The listing builds one solid part. Answer for the finished solid, in the listing's coordinates (mm). A direction names the side the tool comes from. Round coordinates to 2 decimals unless told otherwise and drop trailing zeros. Order: outer loops, then holes, each group sorted by start corner. A loop starts at its lowest first (then second) coordinate and runs counter-clockwise, first axis right, second up. Notation, with made-up numbers: (9, 18.25) - (16, 18.25) arc R8 cw to (16, 27.25) - close; hole circle Ø5 at (24, 80.25). An arc over 180 degrees is marked (long way). One line per item, written item: value. Start each with the question number.
1. A tool of negligible diameter and unlimited length cuts with its end or side. For faces 1 (the cylindrical face through (3.75, 66.42, 4.53)), 2 (the flat face through (30, 70, 2)), 3 (the flat face through (11, 72, 3)), from which of +Z, -Z, +X, -X, +Y, -Y can it reach the whole face along a straight path? Write none if from no direction.
2. Section C-C, the plane x = 10 is taken. Give the vertices of the cut face in (y, z).
3. Section B-B, the plane x = 23.5 is taken. Give the vertices of the cut face in (y, z), then the cut area to 3 significant figures.
4. Section A-A, the plane y = 60 is taken. Give the vertices of the cut face in (x, z).
5. For a pull along Y with two mould halves and no side action, classify faces 4 (the flat face through (1, 66, 2)), 5 (the flat face through (22, 24, 5)), 6 (the flat face through (22, 131, 3)) as released by +Y, released by -Y, zero draft, split by the parting line, or undercut.
6. Straight lines are drawn through the part: line 1 (X direction, y = 39, z = 0.75); line 2 (Y direction, x = 32, z = 3.25); line 3 (Y direction, x = 24, z = 3.75). For each, find the intervals that lie inside material, in ascending order.
7. Flat-ended cylindrical pins translate along their axes: P1, Ø0.6, axis at y = 118, z = 4.5, coming from the -X side; P2, Ø12, axis at x = 32, y = 62, coming from the +Z side; P3, Ø5, axis at x = 27, y = 85, coming from the +Z side; P4, Ø1.6, axis at y = 24.5, z = 4, coming from the -X side. Find the tip coordinate at first contact, or state that the pin passes through.
from build123d import *

# Parameters (mm, degrees)
F0_W      = 45
F0_H      = 131
F1_DEPTH  = 2
F2_W      = 40.5
F2_H      = 131
F3_DEPTH  = 5
F5_W      = 35
F5_H      = 100
F6_DEPTH  = 4
F7_W      = 5
F7_H      = 100
F8_DEPTH  = 2
F4_W      = 15
F4_H      = 90
F9_DEPTH  = 7.001
F10_R     = 1.5
F11_DEPTH = 131.001


with BuildPart() as f1:
    # F0 (on Top) → F1 (new body)
    with BuildSketch(Plane.XY):
        with Locations((22.5, 65.5)):
            Rectangle(F0_W, F0_H)
    extrude(amount=F1_DEPTH)

    # F2 (on face) → F3 (join)
    with BuildSketch(Plane.XY.offset(2)):
        with Locations((22.5, 65.5)):
            Rectangle(F2_W, F2_H)
    extrude(amount=F3_DEPTH)

    # F5 (on face) → F6 (cut)
    with BuildSketch(Plane.XY.offset(7)):
        with Locations((22.5, 71)):
            Rectangle(F5_W, F5_H)
    extrude(amount=-F6_DEPTH, mode=Mode.SUBTRACT)

    # F7 (on face) → F8 (join)
    with BuildSketch(Plane.XY.offset(3)):
        with Locations((22.5, 71)):
            Rectangle(F7_W, F7_H)
    extrude(amount=F8_DEPTH)

    # F4 (on face) → F9 (cut, through all)
    with BuildSketch(Plane.XY.offset(7)):
        with Locations((22.5, 71)):
            Rectangle(F4_W, F4_H)
    extrude(amount=-F9_DEPTH, mode=Mode.SUBTRACT)

    # F10 (on face) → F11 (cut, through all)
    with BuildSketch(Plane(origin=(0, 131, 0), x_dir=(-1, 0, 0), z_dir=(0, 1, 0))):
        with Locations((-42.75, 4.5)):
            Circle(F10_R)
        with Locations((-2.25, 4.5)):
            Circle(F10_R)
    extrude(amount=-F11_DEPTH, mode=Mode.SUBTRACT)


solid = f1.part
Answer list:
1. face 1: -X, +Y, -Y
1. face 2: +Z, -Z
1. face 3: +Z
2. outline: (0, 0) - (131, 0) - (131, 7) - (121, 7) - (121, 3) - (21, 3) - (21, 7) - (0, 7) - close
3. outline: (0, 0) - (26, 0) - (26, 5) - (21, 5) - (21, 7) - (0, 7) - close; (116, 0) - (131, 0) - (131, 7) - (121, 7) - (121, 5) - (116, 5) - close
3. area: 267 mm²
4. outline: (0, 0) - (15, 0) - (15, 3) - (5, 3) - (5, 7) - (2.25, 7) - (2.25, 6) arc R1.5 cw to (2.25, 3) - (2.25, 2) - (0, 2) - close; (30, 0) - (45, 0) - (45, 2) - (42.75, 2) - (42.75, 3) arc R1.5 cw to (42.75, 6) - (42.75, 7) - (40, 7) - (40, 3) - (30, 3) - close
5. face 4: zero draft
5. face 5: undercut
5. face 6: released by +Y
6. line 1: x = 0 to 15, 30 to 45
6. line 2: y = 0 to 21, 121 to 131
6. line 3: y = 0 to 26, 116 to 131
7. P1: stops at x = 3.72
7. P2: stops at z = 3
7. P3: passes through
7. P4: stops at x = 3
